Check sheet for the modelled part. Datum: model origin and axes. Units: mm. A direction names the side the tool comes from. Coordinates: 2 decimals unless noted, no trailing zeros. Use one line per item in the form item = value.
from build123d import *

# Parameters (mm, degrees)
SKETCH1_R                    = 177.8
SKETCH1_R_2                  = 149.225
BOSS_EXTRUDE1_DEPTH          = 28.448
SKETCH2_R                    = 152.654
CUT_EXTRUDE1_DEPTH           = 15.748
CHAMFER1_SIZE                = 0.762
SKETCH3_R                    = 4.953
CUT_EXTRUDE2_DEPTH           = 29.448
CHAMFER2_SIZE                = 0.381
CIRPATTERN1_COUNT            = 30
CHAMFER2_OF_CIRPATTERN1_SIZE = 0.381
CUT_EXTRUDE3_DEPTH           = 0.381


with BuildPart() as part:
    # Sketch1 → Boss-Extrude1 (new body)
    with BuildSketch(Plane(origin=(0, 0, 0), x_dir=(1, 0, 0), z_dir=(0, 1, 0))):
        Circle(SKETCH1_R)
        Circle(SKETCH1_R_2, mode=Mode.SUBTRACT)
    extrude(amount=BOSS_EXTRUDE1_DEPTH)

    # Sketch2 → Cut-Extrude1 (cut)
    with BuildSketch(Plane(origin=(0, 28.448, 0), x_dir=(-1, 0, 0), z_dir=(0, -1, 0))):
        Circle(SKETCH2_R)
    extrude(amount=CUT_EXTRUDE1_DEPTH, mode=Mode.SUBTRACT)

    # Chamfer1
    chamfer1_edges = [part.edges().sort_by_distance(p)[0] for p in [
        (152.654, 28.448, 0),
        (-177.8, 0, 0),
        (-177.8, 28.448, 0),
    ]]
    chamfer(chamfer1_edges, length=CHAMFER1_SIZE)

    # Sketch4 → Cut-Revolve1 (revolve, cut)
    with BuildSketch(Plane.XY):
        Polygon((-156.845, 0), (-156.845, 1.816005512), (-153.67, 0.6604), (-153.67, 1.27), (0, 1.27), (0, 0), align=None)
    revolve(axis=Axis((0, 28.448, 0), (0, -1, 0)), mode=Mode.SUBTRACT)

    # Sketch3 → Cut-Extrude2 (cut, through all)
    with BuildSketch(Plane(origin=(0, 28.448, 0), x_dir=(1, 0, 0), z_dir=(0, 1, 0))):
        with Locations((0, 162.687)):
            Circle(SKETCH3_R)
    cut_extrude2 = extrude(amount=-CUT_EXTRUDE2_DEPTH, mode=Mode.SUBTRACT)

    # Chamfer2
    chamfer2_edges = [part.edges().sort_by_distance(p)[0] for p in [
        (-4.953, 0, -162.687),
        (-4.953, 28.448, -162.687),
    ]]
    chamfer(chamfer2_edges, length=CHAMFER2_SIZE)

    # CirPattern1: Cut-Extrude2 ×30 about axis
    cirpattern1_axis = Axis((0, 0, 0), (0, 1, 0))
    for i in range(1, CIRPATTERN1_COUNT):
        add(cut_extrude2.rotate(cirpattern1_axis, i * 360 / CIRPATTERN1_COUNT), mode=Mode.SUBTRACT)

    # Chamfer2 of CirPattern1
    chamfer2_of_cirpattern1_edges = [part.edges().sort_by_distance(p)[0] for p in [
        (-38.669294311, 0, -158.102112116),
        (-38.669294311, 28.448, -158.102112116),
        (-70.695554904, 0, -146.607403274),
        (-70.695554904, 28.448, -146.607403274),
        (-99.632080513, 0, -128.705247409),
        (-99.632080513, 28.448, -128.705247409),
        (-124.214206116, 0, -105.178054636),
        (-124.214206116, 28.448, -105.178054636),
        (-143.367574865, 0, -77.054076175),
        (-143.367574865, 28.448, -77.054076175),
        (-156.25509264, 0, -45.562464839),
        (-156.25509264, 28.448, -45.562464839),
        (-162.31351307, 0, -12.079555156),
        (-162.31351307, 28.448, -12.079555156),
        (-161.278054113, 0, 21.931289051),
        (-161.278054113, 28.448, 21.931289051),
        (-153.193970293, 0, 54.983630689),
        (-153.193970293, 28.448, 54.983630689),
        (-138.414574865, 0, 85.632923825),
        (-138.414574865, 28.448, 85.632923825),
        (-117.585798329, 0, 112.539647277),
        (-117.585798329, 28.448, 112.539647277),
        (-91.617958167, 0, 134.527848118),
        (-91.617958167, 28.448, 134.527848118),
        (-61.6459736, 0, 150.636536461),
        (-61.6459736, 28.448, 150.636536461),
        (-28.979764178, 0, 160.161685325),
        (-28.979764178, 28.448, 160.161685325),
        (4.953, 0, 162.687),
        (4.953, 28.448, 162.687),
        (38.669294311, 0, 158.102112116),
        (38.669294311, 28.448, 158.102112116),
        (70.695554904, 0, 146.607403274),
        (70.695554904, 28.448, 146.607403274),
        (99.632080513, 0, 128.705247409),
        (99.632080513, 28.448, 128.705247409),
        (124.214206116, 0, 105.178054636),
        (124.214206116, 28.448, 105.178054636),
        (143.367574865, 0, 77.054076175),
        (143.367574865, 28.448, 77.054076175),
        (156.25509264, 0, 45.562464839),
        (156.25509264, 28.448, 45.562464839),
        (162.31351307, 0, 12.079555156),
        (162.31351307, 28.448, 12.079555156),
        (161.278054113, 0, -21.931289051),
        (161.278054113, 28.448, -21.931289051),
        (153.193970293, 0, -54.983630689),
        (153.193970293, 28.448, -54.983630689),
        (138.414574865, 0, -85.632923825),
        (138.414574865, 28.448, -85.632923825),
        (117.585798329, 0, -112.539647277),
        (117.585798329, 28.448, -112.539647277),
        (91.617958167, 0, -134.527848118),
        (91.617958167, 28.448, -134.527848118),
        (61.6459736, 0, -150.636536461),
        (61.6459736, 28.448, -150.636536461),
        (28.979764178, 0, -160.161685325),
        (28.979764178, 28.448, -160.161685325),
    ]]
    chamfer(chamfer2_of_cirpattern1_edges, length=CHAMFER2_OF_CIRPATTERN1_SIZE)

    # Sketch5 → Cut-Extrude3 (cut, symmetric)
    with BuildSketch(Plane.XY):
        Polygon((-155.45787474, 0.893727035), (-177.8, 2.064628205), (-177.8, -7.253474952), (-155.45787474, -7.253474952), align=None)
        Polygon((155.45787474, 0.893727035), (155.45787474, -7.253474952), (177.8, -7.253474952), (177.8, 2.064628205), align=None)
    extrude(amount=CUT_EXTRUDE3_DEPTH, both=True, mode=Mode.SUBTRACT)


solid = part.part
(1) Go/stop test with flat-tipped pins: P1, Ø12, axis at x = -5.5, z = 140, coming from the +Y side; P2, Ø1.5, axis at y = 22, z = -44.5, coming from the -X side; P3, Ø1.5, axis at x = -14, y = 23.5, coming from the +Z side; P4, Ø3, axis at y = 18, z = -7, coming from the +X side. Record where each tip stops, or that it passes through.
Established:
P1 = through
P2 = -172.33
P3 = 177.31
P4 = 177.71
(2) Scan lines: line 1 along Z through (x, y) = (0, 21.75); line 2 along Z through (x, y) = (97, 26.75); line 3 along X through (y, z) = (11.5, 61.5). Record each from-to range of solid material in increasing order.
Established:
line_1 = -177.8 to -167.64, -157.73 to -152.65, 152.65 to 157.73, 167.64 to 177.8
line_2 = -149.01 to -136.37, -126.86 to -117.87, 117.87 to 126.86, 136.37 to 149.01
line_3 = -166.83 to -135.96, 135.96 to 166.83
(3) Section check A-A, the plane x = 0. Give the number of separate pieces and of enclosed holes in the cut face, plus the area to 3 significant figures.
Established:
separate_pieces = 4
enclosed_holes = 0
area = 933 mm²
(4) Tool access check on faces 1 (the cylindrical face through (-136.3, 14.4, 83.2)), 2 (the cylindrical face through (-82.066, 20.298, -128.718)). Record the directions out of +Z, -Z, +X, -X, +Y, -Y that give a thin tool (end or side, any length) a straight path to the whole face; none if there is none.
Established:
face_1 = +Y, -Y
face_2 = +Y
